from build123d import *

# Parameters (mm, degrees)
SKETCH1_W             = 6
SKETCH1_H             = 6
BOSS_EXTRUDE1_DEPTH   = 3
SKETCH2_R             = 1.75
BOSS_EXTRUDE2_DEPTH   = 1.5
SKETCH3_R             = 0.65
BOSS_EXTRUDE3_DEPTH   = 0.5
SKETCH4_W             = 0.64
SKETCH4_H             = 0.64
BOSS_EXTRUDE4_DEPTH   = 3.2
BOSS_EXTRUDE4_2_DEPTH = 3.2
BOSS_EXTRUDE4_3_DEPTH = 3.2
BOSS_EXTRUDE4_4_DEPTH = 3.2
FILLET1_R             = 0.4
SKETCH6_W             = 0.64
SKETCH6_H             = 0.64
BOSS_EXTRUDE6_DEPTH   = 8.26


with BuildPart() as part:
    # Sketch1 → Boss-Extrude1 (new body)
    with BuildSketch(Plane(origin=(0, 0, 0), x_dir=(1, 0, 0), z_dir=(0, 1, 0))):
        Rectangle(SKETCH1_W, SKETCH1_H)
    extrude(amount=BOSS_EXTRUDE1_DEPTH)

    # Sketch2 → Boss-Extrude2 (add)
    with BuildSketch(Plane(origin=(0, 3, 0), x_dir=(1, 0, 0), z_dir=(0, 1, 0))):
        Circle(SKETCH2_R)
    extrude(amount=BOSS_EXTRUDE2_DEPTH)

    # Sketch3 → Boss-Extrude3 (add)
    with BuildSketch(Plane(origin=(0, 3, 0), x_dir=(1, 0, 0), z_dir=(0, 1, 0))):
        with Locations((-2, 2)):
            Circle(SKETCH3_R)
        with Locations((-2, -2)):
            Circle(SKETCH3_R)
        with Locations((2, -2)):
            Circle(SKETCH3_R)
        with Locations((2, 2)):
            Circle(SKETCH3_R)
    extrude(amount=BOSS_EXTRUDE3_DEPTH)

    # Fillet1
    fillet1_edges = [part.edges().sort_by_distance(p)[0] for p in [
        (3, 1.5, 3),
        (-3, 1.5, 3),
        (-3, 1.5, -3),
        (3, 1.5, -3),
    ]]
    fillet(fillet1_edges, radius=FILLET1_R)



with BuildPart() as body_2:
    # Sketch4 → Boss-Extrude4 (new body)
    with BuildSketch(Plane.XZ):
        with Locations((-3.81, 2.54)):
            Rectangle(SKETCH4_W, SKETCH4_H)
    extrude(amount=BOSS_EXTRUDE4_DEPTH)


with BuildPart() as body_3:
    # Sketch4 → Boss-Extrude4 2 (new body)
    with BuildSketch(Plane.XZ):
        with Locations((3.81, 2.54)):
            Rectangle(SKETCH4_W, SKETCH4_H)
    extrude(amount=BOSS_EXTRUDE4_2_DEPTH)


with BuildPart() as body_4:
    # Sketch4 → Boss-Extrude4 3 (new body)
    with BuildSketch(Plane.XZ):
        with Locations((3.81, -2.54)):
            Rectangle(SKETCH4_W, SKETCH4_H)
    extrude(amount=BOSS_EXTRUDE4_3_DEPTH)


with BuildPart() as body_5:
    # Sketch4 → Boss-Extrude4 4 (new body)
    with BuildSketch(Plane.XZ):
        with Locations((-3.81, -2.54)):
            Rectangle(SKETCH4_W, SKETCH4_H)
    extrude(amount=BOSS_EXTRUDE4_4_DEPTH)


with BuildPart() as part_1:
    add(part.part)

    add(body_2.part)  # Boss-Extrude6 merges body 2

    add(body_3.part)  # Boss-Extrude6 merges body 3

    add(body_4.part)  # Boss-Extrude6 merges body 4

    add(body_5.part)  # Boss-Extrude6 merges body 5
    # Sketch6 → Boss-Extrude6 (add)
    with BuildSketch(Plane.ZY.offset(4.13)):
        with Locations((-2.54, 0.32)):
            Rectangle(SKETCH6_W, SKETCH6_H)
        with Locations((2.54, 0.32)):
            Rectangle(SKETCH6_W, SKETCH6_H)
    extrude(amount=-BOSS_EXTRUDE6_DEPTH)


solid = part_1.part
Read the model definition and answer for the solid it produces. Units are mm, in the model's axes. A direction names the side the tool comes from. Coordinates: 2 decimals unless noted, no trailing zeros. Order: outer loops, then holes, each group sorted by start corner. A loop starts at its lowest first (then second) coordinate and runs counter-clockwise, first axis right, second up. Notation, with made-up numbers: (-6.75, 47.25) - (46.25, 47.25) arc R32 cw to (46.25, 76.25) - close; hole circle Ø1 at (59.5, 37.5). An arc over 180 degrees is marked (long way). Use one line per item in the form item = value.
(1) Section B-B, the plane z = 0 is taken. Give the vertices of the cut face in (x, y).
Computed values:
outline = (-3, 0) - (3, 0) - (3, 3) - (1.75, 3) - (1.75, 4.5) - (-1.75, 4.5) - (-1.75, 3) - (-3, 3) - close
(2) Section C-C, the plane y = 0.75 is taken. Give the vertices of the cut face in (x, z), then the cut area to 3 significant figures.
Computed values:
outline = (-3, -2.6) arc R0.4 ccw to (-2.6, -3) - (2.6, -3) arc R0.4 ccw to (3, -2.6) - (3, 2.6) arc R0.4 ccw to (2.6, 3) - (-2.6, 3) arc R0.4 ccw to (-3, 2.6) - close
area = 35.9 mm²
(3) Which of the six approach directions +Z, -Z, +X, -X, +Y, -Y give full straight-line access (tool end or side, diameter ignored) to faces 4 (the face through (-2, 3.5, -2)), 5 (the face through (-3.8, -1.3, 2.22)), 6 (the face through (-3.8, -1.3, -2.86))?
Computed values:
face_4 = -Z, -X, +Y
face_5 = -X, +Y, -Y
face_6 = -Z, -X, +Y, -Y
(4) Straight lines are drawn through the part: L1, parallel to X at y = -0.25, z = -2.55; L2, parallel to Y at x = -2, z = -1.15; L3, parallel to X at y = 1, z = -1.85. For each, find the intervals that lie inside material, in ascending order.
Computed values:
L1 = -4.13 to -3.49, 3.49 to 4.13
L2 = 0 to 3
L3 = -3 to 3
(5) Section D-D, the plane z = -1.6 is taken. Give the vertices of the cut face in (x, y), then the cut area to 3 significant figures.
Computed values:
outline = (-3, 0) - (3, 0) - (3, 3) - (2.51, 3) - (2.51, 3.5) - (1.49, 3.5) - (1.49, 3) - (0.71, 3) - (0.71, 4.5) - (-0.71, 4.5) - (-0.71, 3) - (-1.49, 3) - (-1.49, 3.5) - (-2.51, 3.5) - (-2.51, 3) - (-3, 3) - close
area = 21.2 mm²
(6) For a pull along Z with two mould halves and no side action, classify faces 1 (the face through (3.8, -1.3, 2.86)), 2 (the face through (3.8, -1.3, -2.86)), 3 (the face through (-2.141, 3.246, -1.365)) as pulls with the +Z half, pulls with the -Z half, needs draft (parallel to the pull), parting line crosses it, or undercut.
Computed values:
face_1 = pulls with the +Z half
face_2 = pulls with the -Z half
face_3 = undercut
(7) Section A-A, the plane x = 2 is taken. Give the vertices of the cut face in (y, z), then the cut area to 3 significant figures.
Computed values:
outline = (0, -3) - (3, -3) - (3, -2.65) - (3.5, -2.65) - (3.5, -1.35) - (3, -1.35) - (3, 1.35) - (3.5, 1.35) - (3.5, 2.65) - (3, 2.65) - (3, 3) - (0, 3) - close
area = 19.3 mm²
(8) Given pin 1 Ø1.5 at (y, z) = (2, -1) entering from +X; pin 2 Ø0.9 at (y, z) = (1.5, 0) entering from -X; pin 3 Ø1.2 at (x, y) = (3.5, -1) entering from -Z; pin 4 Ø3 at (x, y) = (-2, -1) entering from +Z, each flat-ended and moving along its own axis, determine where each tip first touches the part or whether it passes through.
Computed values:
pin_1 = 3
pin_2 = -3
pin_3 = -2.86
pin_4 = 3
